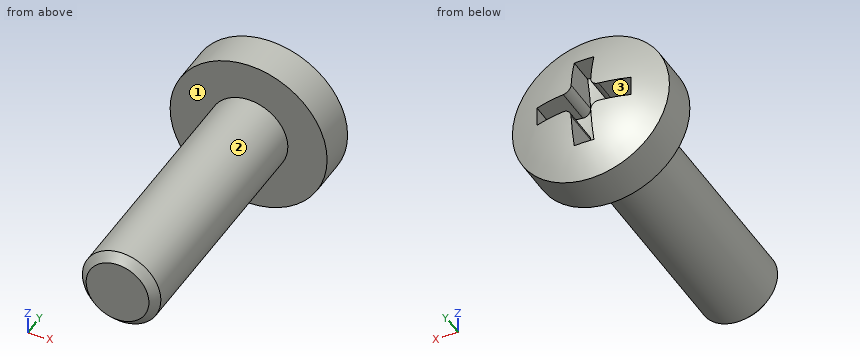
from build123d import *

# Parameters (mm, degrees)
CUT_EXTRUDE1_REACH      = 39.493
CUT_EXTRUDE1_END_RADIUS = 10.625
CUT_EXTRUDE1_START      = 20
FILLET1_R               = 0.5
CHAMFER1_SIZE           = 0.5


with BuildPart() as part:
    # Sketch1 → Revolve1 (revolve)
    with BuildSketch(Plane.XY, mode=Mode.PRIVATE) as revolve1_sk:
        with BuildLine():
            Line((0, 0), (0, 3.8))
            ThreePointArc((0, 3.8), (2.583118271, 3.469685656), (5, 2.5))
            Line((5, 2.5), (5, 0))
            Line((5, 0), (2.5, 0))
            Line((2.5, 0), (2.5, -16))
            Line((2.5, -16), (0, -16))
            Line((0, -16), (0, 0))
        make_face()
    revolve(revolve1_sk.sketch.rotate(Axis((0, 3.8, 0), (0, -1, 0)), 90), axis=Axis((0, 3.8, 0), (0, -1, 0)))

    # Cut-Extrude1: up to this sphere (the profile starts inside it)
    cut_extrude1_end = Location((0, 11.875, 0)) * Sphere(CUT_EXTRUDE1_END_RADIUS, mode=Mode.PRIVATE)
    # Sketch4 → Cut-Extrude1 (cut, up to the surface)
    with BuildSketch(Plane(origin=(0, 0, 0), x_dir=(1, 0, 0), z_dir=(0, 1, 0)).offset(CUT_EXTRUDE1_START), mode=Mode.PRIVATE) as cut_extrude1_sk1:
        Polygon((-0.625, -0.625), (-0.625, -3), (0.625, -3), (0.625, -0.625), (3, -0.625), (3, 0.625), (0.625, 0.625), (0.625, 3), (-0.625, 3), (-0.625, 0.625), (-3, 0.625), (-3, -0.625), align=None)
    cut_extrude1_tool1 = extrude(cut_extrude1_sk1.sketch, amount=-CUT_EXTRUDE1_REACH, mode=Mode.PRIVATE) & cut_extrude1_end
    add(cut_extrude1_tool1.solids().sort_by_distance((0, 20, 0))[0], mode=Mode.SUBTRACT)

    # Fillet1
    fillet1_edges = [part.edges().sort_by_distance(p)[0] for p in [
        (0.625, 2.524352551, 0.625),
        (-0.625, 2.524352551, 0.625),
        (-0.625, 2.524352551, -0.625),
        (0.625, 2.524352551, -0.625),
    ]]
    fillet(fillet1_edges, radius=FILLET1_R)

    # Chamfer1
    chamfer1_edges = [part.edges().sort_by_distance(p)[0] for p in [
        (0, -16, -2.5),
    ]]
    chamfer(chamfer1_edges, length=CHAMFER1_SIZE)


solid = part.part
Geometry: final body of the model. Coordinates: model frame, mm. Face numbers are marked on the shaded views. Coordinates: 2 decimals unless noted, no trailing zeros. Loops run counter-clockwise (first coordinate to the right, second up) from the corner with the lowest first, then second, coordinate; pieces in that order, holes last. Notation, with made-up numbers: (89.25, 62) - (138.25, 62) arc R22 cw to (138.25, 92) - close; hole circle Ø5 at (1, 8). An arc over 180 degrees is marked (long way). Put each result on its own line as item: value. Start each with the question number.
Q1. Cut plane A-A, the plane z = 0. Return loops of the section in (x, y) (3 decimals).
Q2. Cut plane C-C, the plane y = -0.25. Return loops of the section in (x, z), and give its area (3 significant figures).
Q3. Line query: line 1 (X direction, y = -4, z = -1.5); line 2 (X direction, y = 0.5, z = -4); line 3 (Y direction, x = -4, z = 0). Output: solid intervals per line, ascending.
Q4. Pull-direction query (Z, two-part tool) for the marked faces 1, 2 and 3; classes: released by +Z, released by -Z, zero draft, split by the parting line, or undercut.
Q5. Pin query (flat end, axial travel): pin 1 Ø0.6 at (x, y) = (2, 2.5) entering from +Z; pin 2 Ø0.6 at (y, z) = (2, 2.5) entering from -X; pin 3 Ø1 at (x, z) = (0.5, -0.5) entering from +Y; pin 4 Ø5 at (x, y) = (2.5, -3.5) entering from -Z. Return the tip coordinate at first contact, or that it passes through.
Q6. Cut plane D-D, the plane z = 3.5. Return loops of the section in (x, y).
Q7. Cut plane B-B, the plane x = 0. Return loops of the section in (y, z) (3 decimals).
Filled sheet:
1. outline: (-5, 0) - (-2.5, 0) - (-2.5, -15.5) - (-2, -16) - (2, -16) - (2.5, -15.5) - (2.5, 0) - (5, 0) - (5, 2.5) arc R10.265 ccw to (3, 3.352) - (3, 1.682) arc R10.625 cw to (-3, 1.682) - (-3, 3.352) arc R10.265 ccw to (-5, 2.5) - close
2. outline: circle Ø5 at (0, 0)
2. area: 19.6 mm²
3. line 1: -2 to 2
3. line 2: -3 to 3
3. line 3: 0 to 2.99
4. face 1: zero draft
4. face 2: split by the parting line
4. face 3: undercut
5. pin 1: z = 4.7
5. pin 2: x = -4.49
5. pin 3: y = 3.74
5. pin 4: z = -2.5
6. outline: (-3.57, 0) - (3.57, 0) - (3.57, 2.5) arc R9.65 ccw to (-3.57, 2.5) - close
7. outline: (-16, -2) - (-15.5, -2.5) - (0, -2.5) - (0, -5) - (2.5, -5) arc R10.265 ccw to (3.352, -3) - (1.682, -3) arc R10.625 cw to (1.682, 3) - (3.352, 3) arc R10.265 ccw to (2.5, 5) - (0, 5) - (0, 2.5) - (-15.5, 2.5) - (-16, 2) - close
